Verification items for the finished model (mm, model axes). Face numbers are marked on the shaded views. A direction names the side the tool comes from. Coordinates: 2 decimals unless noted, no trailing zeros. Loops run counter-clockwise (first coordinate to the right, second up) from the corner with the lowest first, then second, coordinate; pieces in that order, holes last. Notation, with made-up numbers: (51.5, -30) - (101.5, -30) arc R27 ccw to (101.5, 6) - close; hole circle Ø5 at (72.5, 19). An arc over 180 degrees is marked (long way). Answer as CSV lines item,"result". Start each with the question number.
1. Set-up check for the marked faces 1, 2, 3 and 4: record each of +Z, -Z, +X, -X, +Y, -Y from which the full face is reachable in a straight line by a thin tool's end or side.
2. Cross-section at C-C (z = 15.5). Enter the section's corners in (x, y), plus the area to 3 significant figures.
3. Cross-section at A-A (y = -0.5). Enter the section's corners in (x, z).
4. Cross-section at D-D (x = 11). Enter the section's corners in (y, z).
5. Cross-section at B-B (x = 9.75). Enter the section's corners in (y, z), plus the area to 3 significant figures.
6. Material ranges on line 1 (Z direction, x = 10.75, y = 1.75); line 2 (Z direction, x = 7.25, y = -0.75); line 3 (X direction, y = 0, z = 15.75), recorded low to high. Write a range as [from, to].
7. Gauge pin test, flat ends, axial feed: P1, Ø2.5, axis at y = 0, z = 18, coming from the +X side; P2, Ø1.5, axis at y = 0, z = 17.5, coming from the -X side; P3, Ø1.3, axis at y = 1, z = 15, coming from the -X side. Record the tip position at first contact, or that the pin passes through.
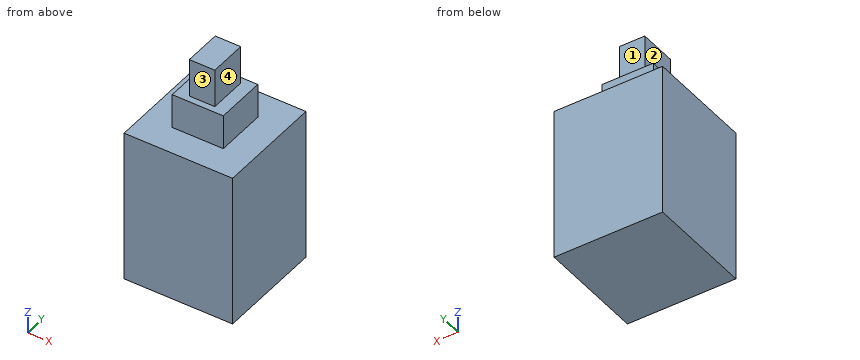
```python
from build123d import *

# Parameters (mm, degrees)
BOX075_W     = 4
BOX075_H     = 4
BOX075_DEPTH = 5.5
BOX076_W     = 8.5
BOX076_H     = 8.5
BOX076_DEPTH = 3.5
BOX078_W     = 2
BOX078_H     = 3
BOX078_DEPTH = 3
BOX074_W     = 8.5
BOX074_H     = 8.5
BOX074_DEPTH = 8.5


with BuildPart() as plunger:
    # Box075 → Box075 (new body)
    with BuildSketch(Plane(origin=(-2, -2, 5.7), x_dir=(1, 0, 0), z_dir=(0, 0, 1))):
        with Locations((2, 2)):
            Rectangle(BOX075_W, BOX075_H)
    extrude(amount=BOX075_DEPTH)


with BuildPart() as pins:
    # Box076 → Box076 (new body)
    with BuildSketch(Plane(origin=(-4.25, -4.25, -3.5), x_dir=(1, 0, 0), z_dir=(0, 0, 1))):
        with Locations((4.25, 4.25)):
            Rectangle(BOX076_W, BOX076_H)
    extrude(amount=BOX076_DEPTH)


with BuildPart() as plunger001:
    # Box078 → Box078 (new body)
    with BuildSketch(Plane(origin=(-1, -1.5, 11.2), x_dir=(1, 0, 0), z_dir=(0, 0, 1))):
        with Locations((1, 1.5)):
            Rectangle(BOX078_W, BOX078_H)
    extrude(amount=BOX078_DEPTH)


with BuildPart() as switch001:
    # Box074 → Box074 (new body)
    with BuildSketch(Plane(origin=(-4.25, -4.25, 0), x_dir=(1, 0, 0), z_dir=(0, 0, 1))):
        with Locations((4.25, 4.25)):
            Rectangle(BOX074_W, BOX074_H)
    extrude(amount=BOX074_DEPTH)

    # Fusion024: union plunger, pins, plunger001
    add(plunger.part)
    add(pins.part)
    add(plunger001.part)


with BuildPart() as switch001_1:
    # Body001 placement: moved
    add(switch001.part.moved(Location((8.5, 0, 5))))


solid = switch001_1.part
```
Values follow:
1,face 1,"+Z, +X, -X, +Y"
1,face 2,"+Z, -X, +Y, -Y"
1,face 3,"+Z, +X, -X, -Y"
1,face 4,"+Z, +X, +Y, -Y"
2,outline,"(6.5, -2) - (10.5, -2) - (10.5, 2) - (6.5, 2) - close"
2,area,"16.0 mm²"
3,outline,"(4.25, 1.5) - (12.75, 1.5) - (12.75, 13.5) - (10.5, 13.5) - (10.5, 16.2) - (9.5, 16.2) - (9.5, 19.2) - (7.5, 19.2) - (7.5, 16.2) - (6.5, 16.2) - (6.5, 13.5) - (4.25, 13.5) - close"
4,outline,"(-4.25, 1.5) - (4.25, 1.5) - (4.25, 13.5) - (-4.25, 13.5) - close"
5,outline,"(-4.25, 1.5) - (4.25, 1.5) - (4.25, 13.5) - (2, 13.5) - (2, 16.2) - (-2, 16.2) - (-2, 13.5) - (-4.25, 13.5) - close"
5,area,"113 mm²"
6,line 1,"z = [1.5, 13.5]"
6,line 2,"z = [1.5, 16.2]"
6,line 3,"x = [6.5, 10.5]"
7,P1,"stops at x = 9.5"
7,P2,"stops at x = 7.5"
7,P3,"stops at x = 6.5"
